The model under review builds one solid part; all positions refer to its coordinate system, in mm. A direction names the side the tool comes from. Coordinates: 2 decimals unless noted, no trailing zeros. Write each loop counter-clockwise with the first axis right and the second up, starting at its lowest first coordinate (ties: lowest second). Pieces come first, ordered by that corner, then holes. Notation, with made-up numbers: (18.25, 4.5) - (30.25, 4.5) arc R37 ccw to (30.25, 40.5) - close; hole circle Ø8 at (55.25, 28.25). An arc over 180 degrees is marked (long way). Return JSON: item names as keys, results as strings. Group by question number.
(1) For pin 1 Ø8 at (x, z) = (-39.5, 226.5) entering from +Y; pin 2 Ø8 at (y, z) = (-15.5, 226) entering from +X; pin 3 Ø2 at (x, z) = (26.5, 62.5) entering from -Y, all flat-tipped, find the tip position at first contact; note any pin that passes through.
(2) To check wall thickness, follow L1, parallel to Z at x = 37, y = -35; L2, parallel to Z at x = -41, y = 8; L3, parallel to Y at x = -0.5, z = 25. State the ranges of each line that lie inside material, in increasing order. Write a range as from..to.
(3) Tool access review of faces 5 (the face through (13.1, -36.2, 337.856)), 6 (the face through (25.841, -19.814, 20.845)), 7 (the face through (-1, 1, 358.247)): name each direction out of +Z, -Z, +X, -X, +Y, -Y from which nothing blocks a thin tool from reaching the whole face with its end or side.
(4) Draft analysis for pull direction Z (two halves, no side actions). For faces 1 (the face through (7.211, 54.924, 347.908)), 2 (the face through (0, 50, 268.011)), 3 (the face through (6.464, 49.234, 251.785)), 4 (the face through (4.298, 32.731, 42.696)), state which applies: released by +Z, released by -Z, zero draft, split by the parting line, or undercut.
(5) We need section A-A on z = 155. State the section outline as (x, y) points, then the cut area to 3 significant figures.
```python
from build123d import *

# Parameters (mm, degrees)
F3_R = 8.434765


with BuildPart() as f2:
    # F1 (on Front) → F2 (revolve)
    with BuildSketch(Plane.XZ):
        Polygon((0, 0), (0, 358.246535), (-55.39559, 358.246535), (-55.39559, 337.855637), (-38.260494, 337.855637), (-38.260494, 295.834184), (-44.670545, 295.834184), (-44.670545, 285.863012), (-66.675, 285.863012), (-66.675, 268.010706), (-49.656138, 268.010706), (-49.656138, 236.007065), (-66.675, 227.296799), (-51.792823, 79.316951), (-41.821633, 72.906896), (-41.821633, 50.827838), (-32.562673, 42.281102), (-32.562673, 0), align=None)
    revolve(axis=Axis((0, 0, 179.123268), (0, 0, -1)))

    # F3
    f3_edges = [f2.edges().sort_by_distance(p)[0] for p in [
        (66.675, 0, 227.296799),
        (51.792823, 0, 79.316951),
    ]]
    fillet(f3_edges, radius=F3_R)


solid = f2.part
```
Ans:
{
 "1": {"pin 1": "y = 55.16", "pin 2": "x = 64.9", "pin 3": "y = -33.15"},
 "2": {"L1": "79.69..235.35, 268.01..285.86, 337.86..358.25", "L2": "50.78..295.83, 337.86..358.25", "L3": "-32.56..32.56"},
 "3": {"face 5": "none", "face 6": "-Z", "face 7": "+Z, +X, -X, +Y, -Y"},
 "4": {"face 1": "zero draft", "face 2": "undercut", "face 3": "undercut", "face 4": "released by -Z"},
 "5": {"outline": "circle Ø118.81 at (0, 0)", "area": "11,100 mm²"}
}
